For this review, take the finished solid that the model builds, in its own axes (mm). A direction names the side the tool comes from. Coordinates: 2 decimals unless noted, no trailing zeros. Loops run counter-clockwise (first coordinate to the right, second up) from the corner with the lowest first, then second, coordinate; pieces in that order, holes last.
1. Machinability: for faces 4 (the face through (2, 0, 6)), 5 (the face through (-2, 24, 6)), 6 (the face through (-1.972, 11.722, 8.998)), 7 (the face through (15, 24, 6)), 8 (the face through (2, 24, 6)), which of the approach directions +Z, -Z, +X, -X, +Y, -Y give a long, thin tool a straight path to every point of the face, cutting with its end or side? Answer none if there is none.
2. To check wall thickness, follow probe 1 along Y at (x, z) = (5.7, 6); probe 2 along Y at (x, z) = (15.5, 9.75). State the ranges of each line that lie inside material, in increasing order.
3. Take a section at C-C, the plane z = 2. State the section outline as (x, y) points.
4. Take a section at D-D, the plane x = -2.5. State the section outline as (y, z) points, then the cut area to 3 significant figures.
5. Take a section at A-A, the plane y = -1.8. State the section outline as (x, z) points, then the cut area to 3 significant figures.
6. Mouldability with a two-part tool opening along Y and no side actions: class faces 1 (the face through (23.054, 22.028, 5.916)), 2 (the face through (5.732, 25.379, 7.016)), 3 (the face through (7, 27.2, 5.9)) as pulls with the +Y half, pulls with the -Y half, needs draft (parallel to the pull), parting line crosses it, or undercut.
7. Take a section at B-B, the plane x = 6. State the section outline as (y, z) points.
8. Clearance check with flat-ended pins moving along their axes: P1, Ø6.5, axis at y = 22, z = 2.5, coming from the -X side; P2, Ø2, axis at x = 3, z = 6.5, coming from the -Y side; P3, Ø5, axis at x = -3.5, y = 12.5, coming from the -Z side; P4, Ø3.5, axis at x = 1, z = 8, coming from the +Y side. State where each tip first meets the part, or that it passes through.
```python
from build123d import *

# Parameters (mm, degrees)
EXTRUDE_1_DEPTH     = 12
SKETCH_3_R          = 1.1
CUT_EXTRUDE_1_DEPTH = 37.558172821
EXTRUDE_2_DEPTH     = 4
SKETCH_11_R         = 2
EXTRUDE_4_DEPTH     = 3.5
CHAMFER_1_SIZE      = 4
CHAMFER_1_SIZE2     = 1.865230633


with BuildPart() as part:
    # 草图1 → 凸台-拉伸1 (new body)
    with BuildSketch(Plane.XY):
        Polygon((7, 24), (7, 28.5), (4.5, 28.5), (4.5, 24), (0, 24), (0, 0), (4.5, 0), (4.5, -4.5), (7, -4.5), (7, 0), (24, 0), (24, 24), align=None)
    extrude(amount=EXTRUDE_1_DEPTH)

    # 草图3 → 切除-拉伸1 (cut, through all)
    with BuildSketch(Plane.ZY.offset(-4.5)):
        with Locations((6, 25.8)):
            Circle(SKETCH_3_R)
        with Locations((6, -1.8)):
            Circle(SKETCH_3_R)
    extrude(amount=-CUT_EXTRUDE_1_DEPTH, mode=Mode.SUBTRACT)

    # 草图10 → 凸台-拉伸2 (add)
    with BuildSketch(Plane.ZY):
        with BuildLine():
            Line((0.984839492, 14.706344723), (5.288002877, 8.154033308))
            ThreePointArc((5.288002877, 8.154033308), (6.054332561, 7.509929186), (6.714260792, 8.262674849))
            Line((6.714260792, 8.262674849), (11.347469324, 15.278865708))
            ThreePointArc((11.347469324, 15.278865708), (5.669013056, 23.990863681), (0.984839492, 14.706344723))
        make_face()
    extrude(amount=EXTRUDE_2_DEPTH)

    # 草图11 → 凸台-拉伸4 (add)
    with BuildSketch(Plane.ZY.offset(4)):
        with Locations((6, 18.8)):
            Circle(SKETCH_11_R)
    extrude(amount=EXTRUDE_4_DEPTH)

    # 倒角1
    chamfer_1_edges = [part.edges().sort_by_distance(p)[0] for p in [
        (24, 24, 6),
    ]]
    chamfer_1_side = [part.faces().sort_by_distance(p)[0] for p in [
        (24, 12, 6),
    ]]
    chamfer(chamfer_1_edges, length=CHAMFER_1_SIZE, length2=CHAMFER_1_SIZE2, reference=chamfer_1_side[0])


solid = part.part
```
Results list:
1. face 4: +Z, -Z, -X, -Y
1. face 5: -X
1. face 6: +Z, -X, -Y
1. face 7: +Z, -Z, +X, +Y
1. face 8: +Z, -Z, -X, +Y
2. probe 1: y = -4.5 to -2.9, -0.7 to 24.7, 26.9 to 28.5
2. probe 2: y = 0 to 24
3. outline: (-4, 13.16) - (0, 13.16) - (0, 0) - (4.5, 0) - (4.5, -4.5) - (7, -4.5) - (7, 0) - (24, 0) - (24, 20) - (22.13, 24) - (7, 24) - (7, 28.5) - (4.5, 28.5) - (4.5, 24) - (0, 24) - (0, 22.47) - (-4, 22.47) - close
4. outline: (8.15, 5.29) - (14.71, 0.98) arc R6 ccw (long way) to (15.28, 11.35) - (8.26, 6.71) arc R0.72 ccw to start
4. area: 132 mm2
5. outline: (4.5, 0) - (7, 0) - (7, 4.9) - (4.5, 4.9) - close; (4.5, 7.1) - (7, 7.1) - (7, 12) - (4.5, 12) - close
5. area: 24.5 mm2
6. face 1: pulls with the +Y half
6. face 2: undercut
6. face 3: needs draft
7. outline: (-4.5, 0) - (28.5, 0) - (28.5, 12) - (-4.5, 12) - close; hole circle Ø2.2 at (-1.8, 6); hole circle Ø2.2 at (25.8, 6)
8. P1: stops at x = -7.5
8. P2: stops at y = 0
8. P3: stops at z = 0.8
8. P4: stops at y = 24
